Source: three-view drawing plus pictorial views. Frame: mm from the lowest corner of the part. A direction names the side the tool comes from. Round coordinates to 2 decimals unless told otherwise and drop trailing zeros. Loops run counter-clockwise (first coordinate to the right, second up) from the corner with the lowest first, then second, coordinate; pieces in that order, holes last. Notation, with made-up numbers: (65, 59.25) -> (105, 59.25) arc R16 cw to (105, 85.25) -> close; hole circle Ø1 at (44.5, 25). An arc over 180 degrees is marked (long way). Answer in a Markdown table with one row per item. Add a question column.
Q1. Ray query, L1, parallel to Z at x = 5, y = 1.55; L2, parallel to Y at x = 3, z = 5.75; L3, parallel to Z at x = 6, y = 1.75. Return the intervals inside material, ascending. Write a range as from..to.
Q2. Mould query, pull axis X, two halves, no side actions, for the marked faces 3, 4 and 5. Classes: pulls with the +X half, pulls with the -X half, needs draft (parallel to the pull), parting line crosses it, or undercut.
Q3. Section C-C, the plane y = 12. Output: boundary loops of the cut face in (x, z), and give its area (3 significant figures).
Q4. Section D-D, the plane z = 3.75. Output: boundary loops of the cut face in (x, y).
Q5. Reachability of the marked faces 1 and 2 from +Z, -Z, +X, -X, +Y, -Y: full face, straight path, thin tool, end or side. Return the list, or none.
Q6. Pin query (flat end, axial travel): pin 1 (3 mm diameter, centred on y = 9, z = 5, fed in from +X); pin 2 (4 mm diameter, centred on x = 5.5, y = 15, fed in from +Z); pin 3 (2 mm diameter, centred on y = 12.5, z = 8.5, fed in from +X). Return the tip coordinate at first contact, or that it passes through.
Q7. Section A-A, the plane z = 5. Output: boundary loops of the cut face in (x, y), and give its area (3 significant figures).
Q8. Section B-B, the plane x = 5. Output: boundary loops of the cut face in (y, z), and give its area (3 significant figures).
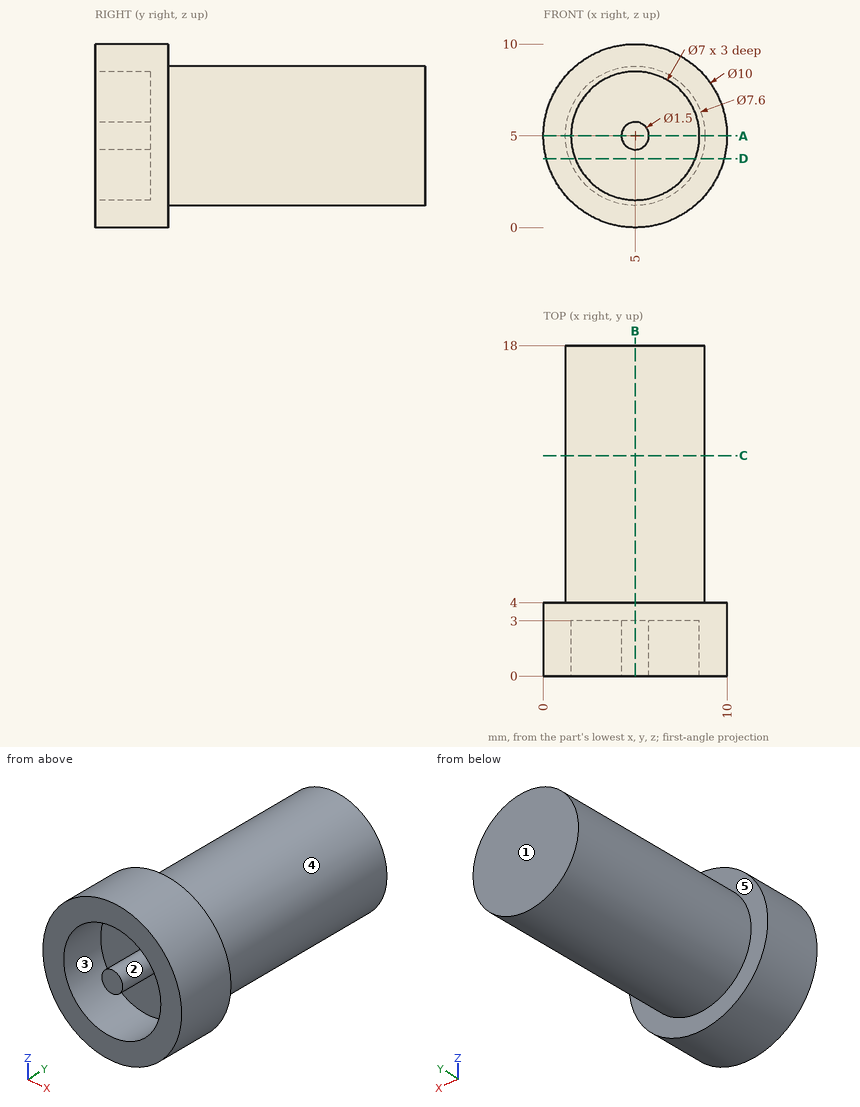
Answer block:
| question | item | result |
|---|---|---|
| 1 | L1 | 0..1.5, 4.25..5.75, 8.5..10 |
| 1 | L2 | 3..18 |
| 1 | L3 | 0.1..1.65, 8.35..9.9 |
| 2 | face 3 | undercut |
| 2 | face 4 | parting line crosses it |
| 2 | face 5 | needs draft |
| 3 | outline | circle Ø7.6 at (5, 5) |
| 3 | area | 45.4 mm^2 |
| 4 | outline | (0.16, 0) -> (1.73, 0) -> (1.73, 3) -> (8.27, 3) -> (8.27, 0) -> (9.84, 0) -> (9.84, 4) -> (8.59, 4) -> (8.59, 18) -> (1.41, 18) -> (1.41, 4) -> (0.16, 4) -> close |
| 5 | face 1 | +Z, -Z, +X, -X, +Y |
| 5 | face 2 | -Y |
| 6 | pin 1 | x = 8.8 |
| 6 | pin 2 | z = 8.8 |
| 6 | pin 3 | x = 7.86 |
| 7 | outline | (0, 0) -> (1.5, 0) -> (1.5, 3) -> (4.25, 3) -> (4.25, 0) -> (5.75, 0) -> (5.75, 3) -> (8.5, 3) -> (8.5, 0) -> (10, 0) -> (10, 4) -> (8.8, 4) -> (8.8, 18) -> (1.2, 18) -> (1.2, 4) -> (0, 4) -> close |
| 7 | area | 130 mm^2 |
| 8 | outline | (0, 0) -> (4, 0) -> (4, 1.2) -> (18, 1.2) -> (18, 8.8) -> (4, 8.8) -> (4, 10) -> (0, 10) -> (0, 8.5) -> (3, 8.5) -> (3, 5.75) -> (0, 5.75) -> (0, 4.25) -> (3, 4.25) -> (3, 1.5) -> (0, 1.5) -> close |
| 8 | area | 130 mm^2 |
